from build123d import *

# Parameters (mm, degrees)
SKETCH_R              = 12
SKETCH_R_2            = 9
PAD_DEPTH             = 39.99
SKETCH001_R           = 11
POCKET_DEPTH          = 7
SKETCH002_R           = 2.1
PAD001_DEPTH          = 10
POLARPATTERN_COUNT    = 3
POCKET001_DEPTH       = 2.5
POLARPATTERN001_COUNT = 3
SKETCH004_R           = 14
SKETCH004_R_2         = 11
PAD002_DEPTH          = 0.01
PAD002_DEPTH_BACK     = 25
CHAMFER_SIZE2         = 5
CHAMFER_SIZE          = 1.99


with BuildPart() as part:
    # Sketch → Pad (new body)
    with BuildSketch(Plane.XY):
        Circle(SKETCH_R)
        Circle(SKETCH_R_2, mode=Mode.SUBTRACT)
    extrude(amount=PAD_DEPTH)

    # Sketch001 (on Face4 of Pad) → Pocket (cut)
    with BuildSketch(Plane.XY.offset(39.99)):
        Circle(SKETCH001_R)
    extrude(amount=-POCKET_DEPTH, mode=Mode.SUBTRACT)

    # Sketch002 (on Face2 of Pocket) → Pad001 (join)
    with BuildSketch(Plane(origin=(0, 0, 0), x_dir=(1, 0, 0), z_dir=(0, 0, -1))):
        with BuildLine():
            Line((-16.52, 6.928203), (-22.52, 3.464102))
            Line((-22.52, 3.464102), (-22.52, -3.464102))
            Line((-22.52, -3.464102), (-16.52, -6.928203))
            Line((-16.52, -6.928203), (-9.797959, -6.928203))
            ThreePointArc((-9.797959, 6.928203), (-12, 0), (-9.797959, -6.928203))
            Line((-16.52, 6.928203), (-9.797959, 6.928203))
        make_face()
        with Locations((-16.52, 0)):
            Circle(SKETCH002_R, mode=Mode.SUBTRACT)
    pad001 = extrude(amount=-PAD001_DEPTH)

    # PolarPattern: Pad001 ×3 about axis
    polarpattern_axis = Axis((0, 0, 0), (0, 0, -1))
    for i in range(1, POLARPATTERN_COUNT):
        add(pad001.rotate(polarpattern_axis, i * 360 / POLARPATTERN_COUNT))

    # Sketch003 (on Face7 of PolarPattern) → Pocket001 (cut, symmetric)
    with BuildSketch(Plane.XY.offset(10)):
        Polygon((-13.02, 2.020726), (-16.52, 4.041452), (-20.02, 2.020726), (-20.02, -2.020726), (-16.52, -4.041452), (-13.02, -2.020726), align=None)
    pocket001 = extrude(amount=POCKET001_DEPTH, both=True, mode=Mode.SUBTRACT)

    # PolarPattern001: Pocket001 ×3 about axis
    polarpattern001_axis = Axis((0, 0, 10), (0, 0, 1))
    for i in range(1, POLARPATTERN001_COUNT):
        add(pocket001.rotate(polarpattern001_axis, i * 360 / POLARPATTERN001_COUNT), mode=Mode.SUBTRACT)

    # Sketch004 (on Face12 of PolarPattern001) → Pad002 (join, two sides)
    with BuildSketch(Plane.XY.offset(39.99)) as pad002_sk:
        Circle(SKETCH004_R)
        Circle(SKETCH004_R_2, mode=Mode.SUBTRACT)
    extrude(amount=PAD002_DEPTH)
    extrude(pad002_sk.sketch, amount=-PAD002_DEPTH_BACK)

    # Chamfer
    chamfer_edges = [part.edges().sort_by_distance(p)[0] for p in [
        (-14, 0, 14.99),
    ]]
    chamfer_side = part.faces().sort_by_distance((-13.60402, 0, 14.99))[0]
    chamfer(chamfer_edges, length=CHAMFER_SIZE, length2=CHAMFER_SIZE2, reference=chamfer_side)


solid = part.part
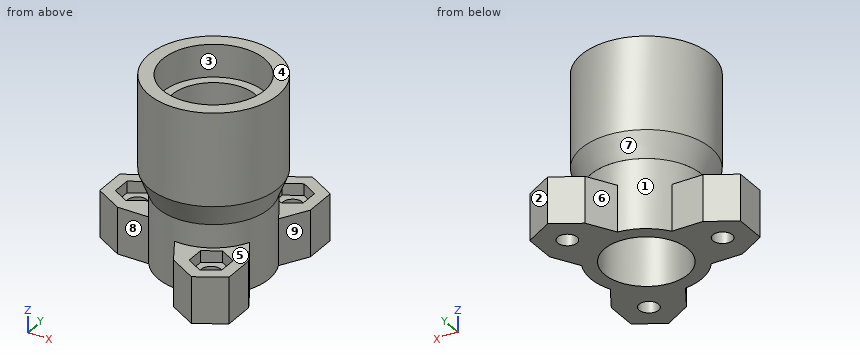
Can you work these out from the model? Positions are in its coordinate system, mm. Face numbers are marked on the shaded views. A direction names the side the tool comes from. Give positions to 0.01 mm unless a question says otherwise; leave off trailing zeros. Order: outer loops, then holes, each group sorted by start corner. A loop starts at its lowest first (then second) coordinate and runs counter-clockwise, first axis right, second up. Notation, with made-up numbers: M -12,-39.75 L 38,-39.75 A8 ccw 38,-26.75 Z; hole C 17.5,-7 d2. An arc over 180 degrees is marked long. Use a Markdown table: item, result. Add a question column.
Item 1: Will these pins go through, and if not, where does the flat tip stop? pin 1 (2 mm diameter, centred on y = -0.5, z = 9, fed in from +X); pin 2 (6 mm diameter, centred on x = 3.5, z = 22.5, fed in from -Y); pin 3 (5 mm diameter, centred on x = -3, z = 9.5, fed in from -Y).
Item 2: For the marked faces 5, 6, 7, 8 and 9, which set-ups out of +Z, -Z, +X, -X, +Y, -Y let a thin tool reach every point of the face, with its end or its side?
Item 3: We'd pull the mould along Y, two halves only. Please class the marked faces 1, 2, 3 and 4: +Y half, -Y half, draft (parallel to the pull), parting line (faces both ways), or undercut.
Item 4: Suppose I cut it at D-D (z = 23.5). List the corners of the cut face in (x, y) for me.
Item 5: Suppose I cut it at B-B (x = -18). List the corners of the cut face in (y, z) for me, then the cut area to 3 significant figures.
Item 6: Suppose I cut it at A-A (y = 0). Count the separate pieces of the cut face and the enclosed holes in it, then the cut area to 3 significant figures.
Item 7: If I drill on L1, parallel to X at y = 0, z = 2.25; L2, parallel to Y at x = 8.26, z = 2; L3, parallel to X at y = 8, z = 33.5, over which ranges is the centre line in solid material (lowest first)? Write a range as [from, to].
Answer sheet:
| question | item | result |
|---|---|---|
| 1 | pin 1 | stops at x = 12 |
| 1 | pin 2 | stops at y = -13.99 |
| 1 | pin 3 | stops at y = -12.99 |
| 2 | face 5 | +X, -Y |
| 2 | face 6 | -Z, -X, +Y |
| 2 | face 7 | none |
| 2 | face 8 | -Z, -X, -Y |
| 2 | face 9 | -Z, +X |
| 3 | face 1 | undercut |
| 3 | face 2 | +Y half |
| 3 | face 3 | undercut |
| 3 | face 4 | draft |
| 4 | outline | C 0,0 d28; hole C 0,0 d18 |
| 5 | outline | M -6.07,0 L -1.49,0 L -1.49,7.5 L -3.19,7.5 L -3.19,10 L -6.07,10 Z; M 1.49,0 L 6.07,0 L 6.07,10 L 3.19,10 L 3.19,7.5 L 1.49,7.5 Z |
| 5 | area | 83.2 mm² |
| 6 | separate pieces | 3 |
| 6 | enclosed holes | 0 |
| 6 | area | 358 mm² |
| 7 | L1 | x = [-22.52, -18.62], [-14.42, -9], [9, 12] |
| 7 | L2 | y = [-21.23, -16.41], [-12.21, -3.57], [3.57, 12.21], [16.41, 21.23] |
| 7 | L3 | x = [-11.49, -7.55], [7.55, 11.49] |
